```python
from build123d import *

# Parameters (mm, degrees)
EXTRUDE_1_DEPTH     = 2
EXTRUDE_1_2_DEPTH   = 0.3
CUT_EXTRUDE_1_REACH = 12.3
SKETCH_3_W          = 2
SKETCH_3_H          = 2


with BuildPart() as part:
    # Эскиз1 → Extrude 1 (new body, symmetric)
    with BuildSketch(Plane.XY):
        with BuildLine():
            Line((-2.480882446, 10), (-2.127329056, 9.646446609))
            ThreePointArc((-2.127329056, 9.646446609), (-1.837573649, 9.0184965), (-2.024597026, 8.352687375))
            ThreePointArc((-2.024597026, 8.352687375), (-2.499401746, 6.831367016), (-1.958507519, 5.332271091))
            ThreePointArc((-1.958507519, 5.332271091), (-1.661010167, 4.685383513), (-1.695318297, 3.974193548))
            ThreePointArc((-1.695318297, 3.974193548), (-2.06411065, 2.399336209), (-2.248797541, 0.79245283))
            ThreePointArc((-2.248797541, 0.79245283), (-2.045132838, 0.234897885), (-1.5, 0))
            Line((-1.5, 0), (0, 0))
            Line((0, 0), (0, -0.3))
            Line((0, -0.3), (-1.5, -0.3))
            ThreePointArc((-1.5, -0.3), (-2.263185974, 0.028857039), (-2.548316557, 0.809433962))
            ThreePointArc((-2.548316557, 0.809433962), (-2.359672091, 2.450750556), (-1.982977044, 4.059354839))
            ThreePointArc((-1.982977044, 4.059354839), (-1.95553054, 4.62830681), (-2.193528422, 5.145816873))
            ThreePointArc((-2.193528422, 5.145816873), (-2.799329956, 6.824804309), (-2.26754867, 8.528683111))
            ThreePointArc((-2.26754867, 8.528683111), (-2.136632306, 8.994749499), (-2.33946109, 9.434314575))
            Line((-2.33946109, 9.434314575), (-2.693014481, 9.787867966))
            Line((-2.693014481, 9.787867966), (-2.480882446, 10))
        make_face()
    extrude_1 = extrude(amount=EXTRUDE_1_DEPTH, both=True)

    # Зеркальное отражение1: Extrude 1 across plane
    add(extrude_1.mirror(Plane(origin=(0, 0, 0), x_dir=(0, 0, 1), z_dir=(1, 0, 0))))

    # Эскиз2 → Extrude 1 2 (add)
    with BuildSketch(Plane.XZ.offset(0.3)):
        Polygon((-1.5, 2), (-1, 2.5), (1, 2.5), (1.5, 2), align=None)
        Polygon((-1.5, -2), (-1, -2.5), (1, -2.5), (1.5, -2), align=None)
    extrude(amount=-EXTRUDE_1_2_DEPTH)

    # Эскиз3 → Вырез-Вытянуть1 (cut, up to next)
    with BuildSketch(Plane.XZ.offset(0.3), mode=Mode.PRIVATE) as cut_extrude_1_sk1:
        Rectangle(SKETCH_3_W, SKETCH_3_H)
    cut_extrude_1_tool1 = extrude(cut_extrude_1_sk1.sketch, amount=-CUT_EXTRUDE_1_REACH, mode=Mode.PRIVATE) & part.part
    add(cut_extrude_1_tool1.solids().sort_by_distance((0, -0.3, 0))[0], mode=Mode.SUBTRACT)


solid = part.part
```
Geometry: final body of the model. Coordinates: model frame, mm. A direction names the side the tool comes from. Coordinates: 2 decimals unless noted, no trailing zeros. Order: outer loops, then holes, each group sorted by start corner. A loop starts at its lowest first (then second) coordinate and runs counter-clockwise, first axis right, second up. Notation, with made-up numbers: (10.5, -26.5) -> (62.5, -26.5) arc R14 ccw to (62.5, -4.5) -> close; hole circle Ø7 at (46, 80.25). An arc over 180 degrees is marked (long way). Write each question's results on one line, items separated by ' | '. Start each with the question number.
1) Material intervals for line 1 along Y through (x, z) = (-1.5, -0.1); line 2 along X through (y, z) = (1.5, -0.7); line 3 along X through (y, z) = (6.5, -0.6), sorted ascending.
2) Set-up query: faces 1 (the cylindrical face through (-2.364, 2.428, 0.028)), 2 (the cylindrical face through (1.84, 9.03, 0.03)), 3 (the cylindrical face through (2.364, 2.428, 0.028)). Return all of +Z, -Z, +X, -X, +Y, -Y with unobstructed straight access to the full face (end or side cutting, diameter ignored); none if empty.
3) Cut plane D-D, the plane z = -1.45. Output: boundary loops of the cut face in (x, y).
4) Cut plane A-A, the plane x = -0.1. Output: boundary loops of the cut face in (y, z).
5) First-contact query: pin 1 (1 mm diameter, centred on x = 2, y = 4.5, fed in from +Z); pin 2 (3 mm diameter, centred on x = 0.5, y = 5.5, fed in from -Z); pin 3 (1.5 mm diameter, centred on x = -0.5, z = -0.5, fed in from +Y); pin 4 (1.5 mm diameter, centred on x = 2, z = -1, fed in from +Y). Flat tips, straight axial feed; report the tip coordinate or a pass-through.
6) Cut plane B-B, the plane y = 3.5. Output: boundary loops of the cut face in (x, z).
Checks:
1) line 1: -0.3 to 0 | line 2: -2.49 to -2.19, 2.19 to 2.49 | line 3: -2.77 to -2.47, 2.47 to 2.77
2) face 1: +Z, -Z, -X | face 2: +Z, -Z | face 3: +Z, -Z, +X
3) outline: (-2.69, 9.79) -> (-2.34, 9.43) arc R0.7 cw to (-2.27, 8.53) arc R2.8 ccw to (-2.19, 5.15) arc R1.2 cw to (-1.98, 4.06) arc R14.3 ccw to (-2.55, 0.81) arc R1.05 ccw to (-1.5, -0.3) -> (1.5, -0.3) arc R1.05 ccw to (2.55, 0.81) arc R14.3 ccw to (1.98, 4.06) arc R1.2 cw to (2.19, 5.15) arc R2.8 ccw to (2.27, 8.53) arc R0.7 cw to (2.34, 9.43) -> (2.69, 9.79) -> (2.48, 10) -> (2.13, 9.65) arc R1 ccw to (2.02, 8.35) arc R2.5 cw to (1.96, 5.33) arc R1.5 ccw to (1.7, 3.97) arc R14 cw to (2.25, 0.79) arc R0.75 cw to (1.5, 0) -> (-1.5, 0) arc R0.75 cw to (-2.25, 0.79) arc R14 cw to (-1.7, 3.97) arc R1.5 ccw to (-1.96, 5.33) arc R2.5 cw to (-2.02, 8.35) arc R1 ccw to (-2.13, 9.65) -> (-2.48, 10) -> close
4) outline: (-0.3, -2.5) -> (0, -2.5) -> (0, -1) -> (-0.3, -1) -> close; (-0.3, 1) -> (0, 1) -> (0, 2.5) -> (-0.3, 2.5) -> close
5) pin 1: z = 2 | pin 2: z = -2 | pin 3: y = 0 | pin 4: y = 10
6) outline: (-2.14, -2) -> (-1.83, -2) -> (-1.83, 2) -> (-2.14, 2) -> close; (1.83, -2) -> (2.14, -2) -> (2.14, 2) -> (1.83, 2) -> close
